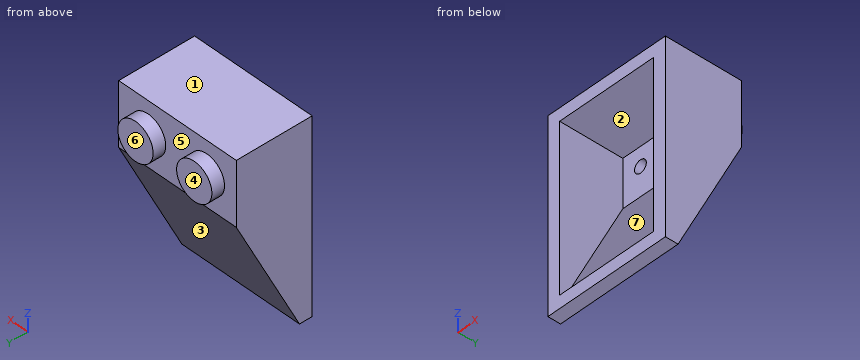
from build123d import *

# Parameters (mm, degrees)
BOSS_EXTRUDE1_DEPTH = 16
SKETCH2_R           = 2.4
BOSS_EXTRUDE2_DEPTH = 1.6
SHELL1_T            = -1.6


with BuildPart() as part:
    # Sketch1 → Boss-Extrude1 (new body)
    with BuildSketch(Plane(origin=(0, 0, 0), x_dir=(0, 0, -1), z_dir=(1, 0, 0))):
        Polygon((0, 0), (24, 0), (24, 1.6), (8, 9.6), (0, 9.6), align=None)
    extrude(amount=BOSS_EXTRUDE1_DEPTH)

    # Sketch2 → Boss-Extrude2 (add)
    with BuildSketch(Plane(origin=(0, 9.6, 0), x_dir=(1, 0, 0), z_dir=(0, 1, 0))):
        with Locations(Location((4, 4, 0), (0, 0, 90))):
            Circle(SKETCH2_R)
        with Locations(Location((12, 4, 0), (0, 0, 90))):
            Circle(SKETCH2_R)
    extrude(amount=BOSS_EXTRUDE2_DEPTH)

    # Shell1
    shell1_openings = [part.faces().sort_by_distance(p)[0] for p in [
        (8, 0, -12),
    ]]
    offset(amount=SHELL1_T, openings=shell1_openings, kind=Kind.INTERSECTION)


solid = part.part
Verification items for the finished model (mm, model axes). Face numbers are marked on the shaded views. A direction names the side the tool comes from. Coordinates: 2 decimals unless noted, no trailing zeros. Loops run counter-clockwise (first coordinate to the right, second up) from the corner with the lowest first, then second, coordinate; pieces in that order, holes last. Notation, with made-up numbers: (23, -21) -> (28, -21) arc R15 ccw to (28, -3) -> close; hole circle Ø3 at (9.5, -24). An arc over 180 degrees is marked (long way). Answer as a JSON object with one key per item and string values. Group by question number.
Item 1: Sectioned sample at B-B on y = 8.75. Record the boundary of the cut face in (x, z).
Item 2: Scan lines: probe 1 along X at (y, z) = (8.7, -4); probe 2 along X at (y, z) = (0.5, -9.5); probe 3 along Y at (x, z) = (8.75, -4.5). Record each from-to range of solid material in increasing order.
Item 3: Sectioned sample at D-D on x = 12. Record the boundary of the cut face in (y, z).
Item 4: Depth check by flat-ended pin: pin 1 (0.8 mm diameter, centred on x = 4.5, z = -4, fed in from -Y); pin 2 (2 mm diameter, centred on x = 5.5, z = -17, fed in from -Y); pin 3 (5 mm diameter, centred on x = 4.5, z = -20, fed in from +Y). Enter the tip coordinate at first touch or a pass-through.
Item 5: Sectioned sample at A-A on x = 8.25. Record the boundary of the cut face in (y, z).
Item 6: Tool access check on the marked faces 5, 6 and 7. Record the directions out of +Z, -Z, +X, -X, +Y, -Y that give a thin tool (end or side, any length) a straight path to the whole face; none if there is none.
Item 7: Mould release check, pull along Z, two halves, no side actions. Record for the marked faces 1, 2, 3 and 4: +Z half, -Z half, draft (parallel to the pull), parting line (faces both ways), or undercut.
Item 8: Sectioned sample at C-C on z = -4. Record the boundary of the cut face in (x, y), plus the area to 3 significant figures.
Evaluation:
{
 "1": {"outline": "(0, -9.7) -> (16, -9.7) -> (16, 0) -> (0, 0) -> close; hole circle Ø1.6 at (4, -4); hole circle Ø1.6 at (12, -4)"},
 "2": {"probe 1": "x = 0 to 3.2, 4.8 to 11.2, 12.8 to 16", "probe 2": "x = 0 to 1.6, 14.4 to 16", "probe 3": "y = 8 to 9.6"},
 "3": {"outline": "(0, -24) -> (1.6, -24) -> (9.6, -8) -> (9.6, -6.4) -> (11.2, -6.4) -> (11.2, -1.6) -> (9.6, -1.6) -> (9.6, 0) -> (0, 0) -> (0, -1.6) -> (8, -1.6) -> (8, -3.2) -> (9.6, -3.2) -> (9.6, -4.8) -> (8, -4.8) -> (8, -7.62) -> (0.61, -22.4) -> (0, -22.4) -> close"},
 "4": {"pin 1": "stops at y = 8", "pin 2": "stops at y = 2.81", "pin 3": "stops at y = 4.85"},
 "5": {"outline": "(0, -24) -> (1.6, -24) -> (9.6, -8) -> (9.6, 0) -> (0, 0) -> (0, -1.6) -> (8, -1.6) -> (8, -7.62) -> (0.61, -22.4) -> (0, -22.4) -> close"},
 "6": {"face 5": "+Y", "face 6": "+Z, -Z, +X, -X, +Y", "face 7": "-Y"},
 "7": {"face 1": "+Z half", "face 2": "undercut", "face 3": "-Z half", "face 4": "draft"},
 "8": {"outline": "(0, 0) -> (1.6, 0) -> (1.6, 8) -> (3.2, 8) -> (3.2, 9.6) -> (4.8, 9.6) -> (4.8, 8) -> (11.2, 8) -> (11.2, 9.6) -> (12.8, 9.6) -> (12.8, 8) -> (14.4, 8) -> (14.4, 0) -> (16, 0) -> (16, 9.6) -> (14.4, 9.6) -> (14.4, 11.2) -> (9.6, 11.2) -> (9.6, 9.6) -> (6.4, 9.6) -> (6.4, 11.2) -> (1.6, 11.2) -> (1.6, 9.6) -> (0, 9.6) -> close", "area": "61.4 mm²"}
}
